Source: CAD feature listing. Evaluate the final solid. Frame: model axes, mm. Coordinates: 2 decimals unless noted, no trailing zeros. Loops run counter-clockwise (first coordinate to the right, second up) from the corner with the lowest first, then second, coordinate; pieces in that order, holes last.
Item 1: Section query C-C, the plane y = 29.5. Return the cut outline in (x, z), then the cut area to 3 significant figures.
Item 2: Section query D-D, the plane x = -17.5. Return the cut outline in (y, z).
Item 3: Section query B-B, the plane z = -19.5. Return the cut outline in (x, y), then the cut area to 3 significant figures.
Item 4: Pin query (flat end, axial travel): pin 1 Ø1.5 at (y, z) = (-39, -2.5) entering from +X; pin 2 Ø12 at (x, z) = (-3, 7) entering from +Y; pin 3 Ø6 at (x, y) = (-14, 71.5) entering from +Z. Return the tip coordinate at first contact, or that it passes through.
Item 5: Section query A-A, the plane x = -3. Return the cut outline in (y, z), then the cut area to 3 significant figures.
Item 6: Line query: probe 1 along Y at (x, z) = (-5.75, -21.5); probe 2 along Z at (x, y) = (-2.25, -47.5); probe 3 along X at (y, z) = (-35, 46). Output: solid intervals per line, ascending.
```python
from build123d import *

# Parameters (mm, degrees)
F0_W     = 195.9732845426
F0_H     = 110.0095510483
F1_DEPTH = 20
F2_R     = 59.148
F4_DEPTH = 8


with BuildPart() as f1:
    # F0 (on Right) → F1 (new body)
    with BuildSketch(Plane.YZ):
        with Locations((-0.1502893865, 0.1502856612)):
            Rectangle(F0_W, F0_H)
    extrude(amount=-F1_DEPTH)

    # F2
    f2_edges = [f1.edges().sort_by_distance(p)[0] for p in [
        (-10, 97.836353, 55.155061),
    ]]
    fillet(f2_edges, radius=F2_R)

    # F3 (on face) → F4 (cut)
    with BuildSketch(Plane.YZ):
        with BuildLine():
            Line((38.6883528848, 47.1550611854), (-98.1369316578, 47.1550611854))
            Line((-98.1369316578, 47.1550611854), (-98.1369316578, 39.1550611854))
            Line((-98.1369316578, 39.1550611854), (38.6883528848, 39.1550611854))
            ThreePointArc((38.6883528848, 39.1550611854), (65.5487139379, 27.2398659264), (76.5687220266, 0))
            Line((76.5687220266, 0), (76.5687220266, -54.8544898629))
            Line((76.5687220266, -54.8544898629), (84.5687220266, -54.8544898629))
            Line((84.5687220266, -54.8544898629), (84.5687220266, 0))
            ThreePointArc((84.5687220266, 0), (71.2059826894, 32.896079052), (38.6883528848, 47.1550611854))
        make_face()
    extrude(amount=-F4_DEPTH, mode=Mode.SUBTRACT)


solid = f1.part
```
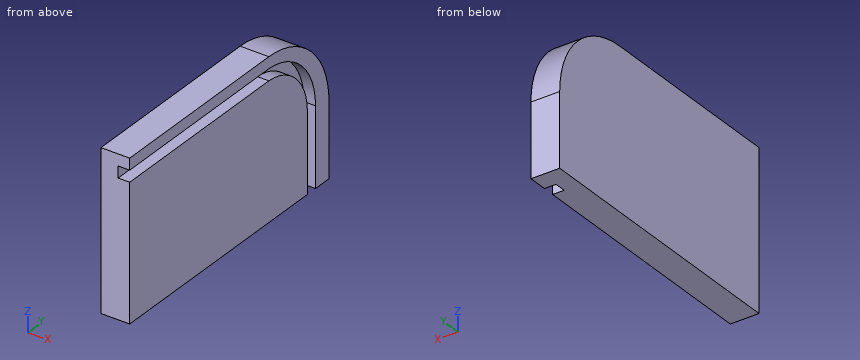
Verdict:
1. outline: (-20, -54.85) - (0, -54.85) - (0, 39.16) - (-8, 39.16) - (-8, 47.16) - (0, 47.16) - (0, 55.16) - (-20, 55.16) - close
1. area: 2,140 mm2
2. outline: (-98.14, -54.85) - (97.84, -54.85) - (97.84, -3.99) arc R59.15 ccw to (38.69, 55.16) - (-98.14, 55.16) - close
3. outline: (-20, -98.14) - (0, -98.14) - (0, 76.57) - (-8, 76.57) - (-8, 84.57) - (0, 84.57) - (0, 97.84) - (-20, 97.84) - close
3. area: 3,860 mm2
4. pin 1: stops at x = 0
4. pin 2: stops at y = 97.63
4. pin 3: stops at z = 47.09
5. outline: (-98.14, -54.85) - (76.57, -54.85) - (76.57, 0) arc R39.18 ccw to (38.69, 39.16) - (-98.14, 39.16) - close; (-98.14, 47.16) - (38.69, 47.16) arc R47.17 cw to (84.57, 0) - (84.57, -54.85) - (97.84, -54.85) - (97.84, -3.99) arc R59.15 ccw to (38.69, 55.16) - (-98.14, 55.16) - close
5. area: 18,700 mm2
6. probe 1: y = -98.14 to 76.57, 84.57 to 97.84
6. probe 2: z = -54.85 to 39.16, 47.16 to 55.16
6. probe 3: x = -20 to -8
